Read the model definition and answer for the solid it produces. Units are mm, in the model's axes. A direction names the side the tool comes from. Coordinates: 2 decimals unless noted, no trailing zeros. Loops run counter-clockwise (first coordinate to the right, second up) from the corner with the lowest first, then second, coordinate; pieces in that order, holes last.
Q1. The mould has two halves that part along Y. Classify faces 3 (the face through (-2, 247.65, -9)), 4 (the face through (9, 254, -1)), 5 (the face through (-2, 125, -127)): pulls with the +Y half, pulls with the -Y half, needs draft (parallel to the pull), parting line crosses it, or undercut.
Q2. Flat-ended cylindrical pins translate along their axes: P1, Ø7.5, axis at x = 0, z = 0, coming from the +Y side; P2, Ø12, axis at x = 37.5, z = -81.5, coming from the -Y side; P3, Ø6, axis at x = 49.5, z = 94.5, coming from the +Y side. Find the tip coordinate at first contact, or state that the pin passes through.
Q3. Section A-A (x = 0) is taken. Give the vertices of the cut face in (y, z) (3 decimals).
Q4. Which of the six approach directions +Z, -Z, +X, -X, +Y, -Y give full straight-line access (tool end or side, diameter ignored) to faces 1 (the face through (-2, 132, -123.825)), 2 (the face through (-2, 125, 127))?
Q5. Section D-D (y = 40) is taken. Give the vertices of the cut face in (x, z) (3 decimals), then the cut area to 3 significant figures.
Q6. Section B-B (z = 0) is taken. Give the vertices of the cut face in (x, y) (3 decimals), then the cut area to 3 significant figures.
Q7. Straight lines are drawn through the part: line 1 (Z direction, x = 0, y = 250) (3 decimals); line 2 (X direction, y = 164.5, z = 6.5) (3 decimals); line 3 (Y direction, x = 54, z = 3.5). For each, find the intervals that lie inside material, in ascending order.
Q8. Section C-C (x = 49) is taken. Give the vertices of the cut face in (y, z) (3 decimals).
from build123d import *

# Parameters (mm, degrees)
SKETCH1_W           = 254
SKETCH1_H           = 254
BOSS_EXTRUDE1_DEPTH = 254
SKETCH2_W           = 247.65
SKETCH2_H           = 247.65
CUT_EXTRUDE1_DEPTH  = 247.65
SKETCH3_R           = 6.35
CUT_EXTRUDE2_DEPTH  = 247.65
SKETCH4_W           = 247.65
SKETCH4_H           = 25.4
SKETCH4_R           = 6.35
BOSS_EXTRUDE2_DEPTH = 6.35


with BuildPart() as part:
    # Sketch1 → Boss-Extrude1 (new body)
    with BuildSketch(Plane(origin=(0, 0, 0), x_dir=(1, 0, 0), z_dir=(0, 1, 0))):
        Rectangle(SKETCH1_W, SKETCH1_H)
    extrude(amount=BOSS_EXTRUDE1_DEPTH)

    # Sketch2 → Cut-Extrude1 (cut)
    with BuildSketch(Plane(origin=(0, 254, 0), x_dir=(1, 0, 0), z_dir=(0, 1, 0))):
        Rectangle(SKETCH2_W, SKETCH2_H)
    extrude(amount=-CUT_EXTRUDE1_DEPTH, mode=Mode.SUBTRACT)

    # Sketch3 → Cut-Extrude2 (cut)
    with BuildSketch(Plane(origin=(0, 6.35, 0), x_dir=(1, 0, 0), z_dir=(0, 1, 0))):
        Circle(SKETCH3_R)
    extrude(amount=-CUT_EXTRUDE2_DEPTH, mode=Mode.SUBTRACT)

    # Sketch4 → Boss-Extrude2 (add)
    with BuildSketch(Plane(origin=(0, 254, 0), x_dir=(1, 0, 0), z_dir=(0, 1, 0))):
        Rectangle(SKETCH4_W, SKETCH4_H)
        Circle(SKETCH4_R, mode=Mode.SUBTRACT)
    extrude(amount=-BOSS_EXTRUDE2_DEPTH)


solid = part.part
Numbers:
1. face 3: undercut
1. face 4: pulls with the +Y half
1. face 5: needs draft
2. P1: passes through
2. P2: stops at y = 0
2. P3: stops at y = 6.35
3. outline: (0, -127) - (254, -127) - (254, -123.825) - (6.35, -123.825) - (6.35, -6.35) - (0, -6.35) - close; (0, 6.35) - (6.35, 6.35) - (6.35, 123.825) - (254, 123.825) - (254, 127) - (0, 127) - close; (247.65, -12.7) - (254, -12.7) - (254, -6.35) - (247.65, -6.35) - close; (247.65, 6.35) - (254, 6.35) - (254, 12.7) - (247.65, 12.7) - close
4. face 1: +Y
4. face 2: +Z, +X, -X, +Y, -Y
5. outline: (-127, -127) - (127, -127) - (127, 127) - (-127, 127) - close; hole (-123.825, -123.825) - (123.825, -123.825) - (123.825, 123.825) - (-123.825, 123.825) - close
5. area: 3,190 mm2
6. outline: (-127, 0) - (-6.35, 0) - (-6.35, 6.35) - (-123.825, 6.35) - (-123.825, 247.65) - (-6.35, 247.65) - (-6.35, 254) - (-127, 254) - close; (6.35, 0) - (127, 0) - (127, 254) - (6.35, 254) - (6.35, 247.65) - (123.825, 247.65) - (123.825, 6.35) - (6.35, 6.35) - close
6. area: 4,600 mm2
7. line 1: z = -127 to -123.825, -12.7 to -6.35, 6.35 to 12.7, 123.825 to 127
7. line 2: x = -127 to -123.825, 123.825 to 127
7. line 3: y = 0 to 6.35, 247.65 to 254
8. outline: (0, -127) - (254, -127) - (254, -123.825) - (6.35, -123.825) - (6.35, 123.825) - (254, 123.825) - (254, 127) - (0, 127) - close; (247.65, -12.7) - (254, -12.7) - (254, 12.7) - (247.65, 12.7) - close
